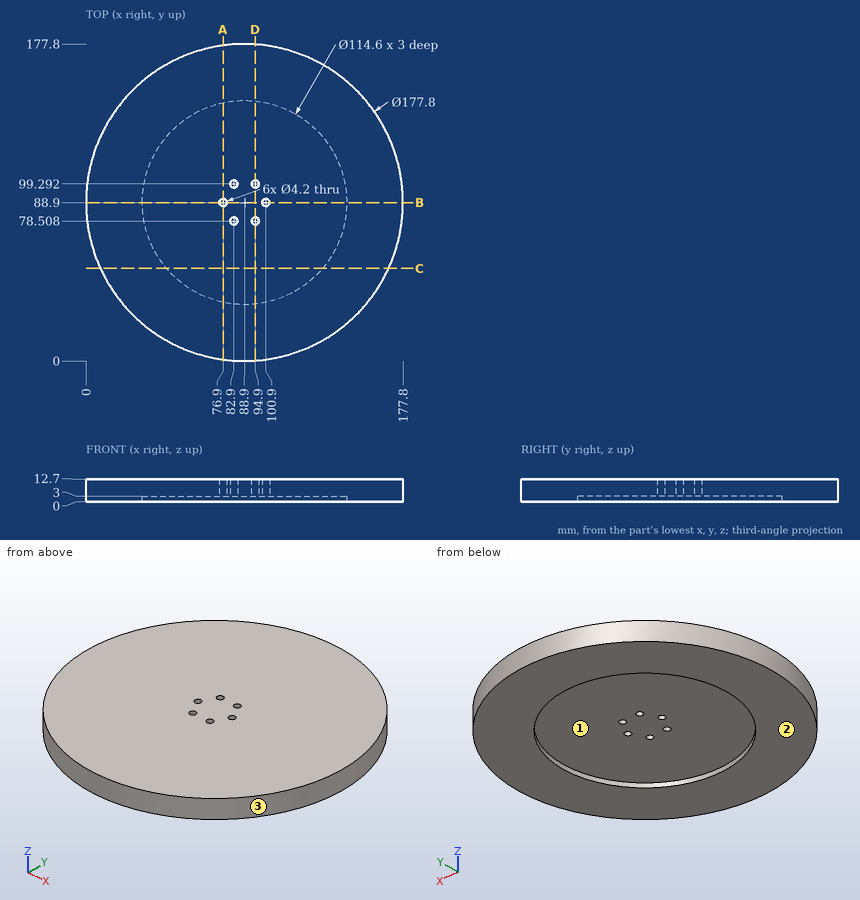
The figure shows three views and two pictorial views of one solid part (mm, origin at its lowest corner). Answer the questions. Coordinates: 2 decimals unless noted, no trailing zeros. Loops run counter-clockwise (first coordinate to the right, second up) from the corner with the lowest first, then second, coordinate; pieces in that order, holes last. Notation, with made-up numbers: (-28.5, 3.25) - (-0.5, 3.25) arc R27 ccw to (-0.5, 19.25) - close; hole circle Ø9 at (-18, 28). An arc over 180 degrees is marked (long way). Use a Markdown table: item, result. Add a question column.
1) Find the intervals of material crossed by line 1 (Y direction, x = 96, z = 9.5) (1 decimal); line 2 (Y direction, x = 88.9, z = 0.95); line 3 (Y direction, x = 82.9, z = 6.25), in increasing order.
2) The part is cut by section D-D, the plane x = 94.9. Give the vertices of the cut face in (y, z) (1 decimal), and give its area (3 significant figures).
3) Given pin 1 (4 mm diameter, centred on x = 94.9, y = 78.51, fed in from +Z); pin 2 (1.5 mm diameter, centred on y = 61.5, z = 8, fed in from -X); pin 3 (5 mm diameter, centred on x = 100.9, y = 88.9, fed in from +Z); pin 4 (1 mm diameter, centred on y = 28.5, z = 1.5, fed in from -X), each flat-ended and moving along its own axis, determine where each tip first touches the part or whether it passes through.
4) The part is cut by section C-C, the plane y = 52. Give the vertices of the cut face in (x, z).
5) The part is cut by section B-B, the plane y = 88.9. Give the vertices of the cut face in (x, z).
6) The part is cut by section A-A, the plane x = 76.9. Give the vertices of the cut face in (y, z).
7) The mould has two halves that part along Y. Classify the marked faces 1, 2 and 3: released by +Y, released by -Y, zero draft, split by the parting line, or undercut.
Here are the results:
| question | item | result |
|---|---|---|
| 1 | line 1 | y = 0.3 to 76.7, 80.3 to 97.5, 101.1 to 177.5 |
| 1 | line 2 | y = 0 to 31.6, 146.2 to 177.8 |
| 1 | line 3 | y = 0.2 to 76.41, 80.61 to 97.19, 101.39 to 177.6 |
| 2 | outline | (0.2, 0) - (31.9, 0) - (31.9, 3) - (76.4, 3) - (76.4, 12.7) - (0.2, 12.7) - close; (80.6, 3) - (97.2, 3) - (97.2, 12.7) - (80.6, 12.7) - close; (101.4, 3) - (145.9, 3) - (145.9, 0) - (177.6, 0) - (177.6, 12.7) - (101.4, 12.7) - close |
| 2 | area | 1,830 mm^2 |
| 3 | pin 1 | passes through |
| 3 | pin 2 | stops at x = 4.09 |
| 3 | pin 3 | stops at z = 12.7 |
| 3 | pin 4 | stops at x = 23.21 |
| 4 | outline | (8.02, 0) - (45.06, 0) - (45.06, 3) - (132.74, 3) - (132.74, 0) - (169.78, 0) - (169.78, 12.7) - (8.02, 12.7) - close |
| 5 | outline | (0, 0) - (31.6, 0) - (31.6, 3) - (74.8, 3) - (74.8, 12.7) - (0, 12.7) - close; (79, 3) - (98.8, 3) - (98.8, 12.7) - (79, 12.7) - close; (103, 3) - (146.2, 3) - (146.2, 0) - (177.8, 0) - (177.8, 12.7) - (103, 12.7) - close |
| 6 | outline | (0.81, 0) - (32.87, 0) - (32.87, 3) - (86.8, 3) - (86.8, 12.7) - (0.81, 12.7) - close; (91, 3) - (144.93, 3) - (144.93, 0) - (176.99, 0) - (176.99, 12.7) - (91, 12.7) - close |
| 7 | face 1 | undercut |
| 7 | face 2 | zero draft |
| 7 | face 3 | split by the parting line |
